Autodesk Inventor part; units mm, degrees
ref_plane "YZ Plane" through (0, 0, 0) normal (1, 0, 0) x (0, 1, 0)
ref_plane "XZ Plane" through (0, 0, 0) normal (0, 1, 0) x (-1, 0, 0)
ref_plane "XY Plane" through (0, 0, 0) normal (0, 0, 1) x (1, 0, 0)
sketch "スケッチ1" plane through (0, 0, 0) normal (0, 1, 0) x (-1, 0, 0)
  circle A0 centre (0, -0.4884) radius 251
  point P0 (0, 0)
  dimension "d0" = 502
extrude "押し出し1" add sketch "スケッチ1" along normal blind 1
sketch "スケッチ2" plane through (0, 1, -0.4884) normal (0, 1, 0) x (1, 0, 0)
  circle A0 centre (0, -0.4884) radius 250
  line L0 (0, -0.4884) -> (-242.4474, -65.4519)
  line L1 (0, -0.4884) -> (251, -0.4884) construction
  line L2 (0, -0.4884) -> (242.4474, -65.4519)
  line L3 (0, -0.4884) -> (251, -0.4884) construction
  line L4 (242.4474, -65.4519) -> (-242.4474, -65.4519)
  circle A1 centre (0, -0.4884) radius 251
  point P0 (242.4474, -65.4519)
  point P1 (-242.4474, -65.4519)
  point P2 (-241.4815, -65.1931)
  point P3 (241.4815, -65.1931)
  dimension "d3" = 500
  dimension "d4" = 251
  dimension "d5" = 165
  dimension "d6" = 251
  dimension "d7" = 15
  dimension "d8" = 502
extrude "押し出し2" add sketch "スケッチ2" along normal blind 200 contours A0 L0 A1 L2
properties part number "stage" material "ステンレス鋼"
Can you work these out from the model? Positions are in its coordinate system, mm. Round coordinates to 2 decimals unless told otherwise and drop trailing zeros. Loops run counter-clockwise (first coordinate to the right, second up) from the corner with the lowest first, then second, coordinate; pieces in that order, holes last. Notation, with made-up numbers: (-3, 53.5) - (12, 53.5) arc R28 ccw to (12, 83.5) - close; hole circle Ø11 at (35.25, -32). An arc over 180 degrees is marked (long way). Use CSV: the item, a comma, the result in double quotes. Start each with the question number.
1) If we section it at C-C on y = 170: Write out the boundary of the cut face in (x, z), plus the area to 3 significant figures.
2) Please list where these lines run through material, in increasing order: probe 1 along X at (y, z) = (71.5, 0); probe 2 along X at (y, z) = (173, -65); probe 3 along Y at (x, z) = (-17.5, 36). Write a range as [from, to].
3) If we section it at B-B on z = -215: Write out the boundary of the cut face in (x, y).
4) For pin 1 Ø5 at (x, y) = (53.5, 116) entering from +Z; pin 2 Ø2 at (y, z) = (126.5, 56.5) entering from +X; pin 3 Ø3 at (x, y) = (60.5, 146) entering from -Z, each with a flat end and sliding along its axis, tell me the tip position at first contact or that it passes through.
5) If we section it at A-A on x = 0: Write out the boundary of the cut face in (y, z), plus the area to 3 significant figures.
6) We'd pull the mould along X, two halves only. Please class faces 1 (the flat face through (4, 0, 3)), 2 (the cylindrical face through (-6.413, 99.6, -249.918)), 3 (the cylindrical face through (250.757, 0.493, -11.524)): released by +X, released by -X, zero draft, split by the parting line, or undercut.
7) If we section it at D-D on x = -190: Write out the boundary of the cut face in (y, z).
Geometry results:
1,outline,"(-242.45, 64.96) arc R251 ccw (long way) to (242.45, 64.96) - (241.48, 64.7) arc R250 cw (long way) to (-241.48, 64.7) - close"
1,area,"918 mm2"
2,probe 1,"x = [-251, -250], [250, 251]"
2,probe 2,"x = [-242.44, -241.4], [241.4, 242.44]"
2,probe 3,"y = [0, 1]"
3,outline,"(-130.33, 0) - (130.33, 0) - (130.33, 1) - (129.52, 1) - (129.52, 201) - (127.57, 201) - (127.57, 1) - (-127.57, 1) - (-127.57, 201) - (-129.52, 201) - (-129.52, 1) - (-130.33, 1) - close"
4,pin 1,"stops at z = -243.65"
4,pin 2,"stops at x = 244.79"
4,pin 3,"stops at z = -243.97"
5,outline,"(0, -251.49) - (1, -251.49) - (1, -251) - (201, -251) - (201, -250) - (1, -250) - (1, 250.51) - (0, 250.51) - close"
5,area,"702 mm2"
6,face 1,"zero draft"
6,face 2,"undercut"
6,face 3,"split by the parting line"
7,outline,"(0, -164.5) - (1, -164.5) - (1, -164.02) - (201, -164.02) - (201, -162.48) - (1, -162.48) - (1, 163.53) - (0, 163.53) - close"
